Check sheet for the modelled part. Datum: model origin and axes. Units: mm. Coordinates: 2 decimals unless noted, no trailing zeros. Write each loop counter-clockwise with the first axis right and the second up, starting at its lowest first coordinate (ties: lowest second). Pieces come first, ordered by that corner, then holes. Notation, with made-up numbers: (-5, 71) - (9, 71) arc R25 cw to (9, 104) - close; hole circle Ø5 at (0, 67). An arc over 180 degrees is marked (long way). Use one line per item in the form item = value. Start each with the question number.
1. Cross-section at A-A on y = 0.25. Record the boundary of the cut face in (x, z).
2. Cross-section at B-B on y = -5. Record the boundary of the cut face in (x, z).
3. Scan lines: line 1 along Y through (x, z) = (-2, -45); line 2 along X through (y, z) = (3.75, -23); line 3 along X through (y, z) = (3.75, -35). Record each from-to range of solid material in increasing order.
4. Cross-section at C-C on y = 5.5. Record the boundary of the cut face in (x, z).
5. Go/stop test with flat-tipped pins: pin 1 Ø10 at (x, z) = (-1.5, -23.5) entering from -Y; pin 2 Ø2 at (y, z) = (-4, -29.5) entering from +X; pin 3 Ø3 at (y, z) = (-2.5, -75.5) entering from -X. Record where each tip stops, or that it passes through.
```python
from build123d import *

# Parameters (mm, degrees)
F1_DEPTH    = 6.35
F2_DEPTH    = 6.35
F4_DEPTH    = 25.4
F5_T1_DEPTH = 66.3794734437
F5_T3_DEPTH = 66.4252991911
F5_T5_DEPTH = 63.2525240866
F5_T7_DEPTH = 63.2028524021


# Not quite as in the source:
# - a fillet or chamfer that OpenCascade refuses, or shapes differently, is made with other operations: its cross-section is extruded or revolved along the edge and cut away or added


with BuildPart() as f1:
    # F0 (on Front) → F1 (new body)
    with BuildSketch(Plane.XZ):
        Polygon((10.5009634349, -8.6313571018), (0, -8.4001217037), (-10.5245159939, -8.168367669), (-8.3013391122, -91.856867075), (8.6683045514, -91.856867075), align=None)
    extrude(amount=F1_DEPTH)

    # F2 (add): a face of the model
    f2_faces = [f1.faces().sort_by_distance(p)[0] for p in [
        (0.0745348421, 0, -48.6438367355),
    ]]
    extrude(f2_faces, amount=F2_DEPTH)

    # F3 (on face) → F4 (cut)
    with BuildSketch(Plane.XZ.offset(6.35)):
        Polygon((7.741477061, -8.5705921125), (0, -12.6956291497), (-8.4089043082, -8.2149542811), (-10.5245159939, -8.168367669), (-10.4707083295, -10.1938847244), (0, -15.2933746576), (10.4665109394, -10.1959289555), (10.5009634349, -8.6313571018), align=None)
        Polygon((-8.4089043082, -8.2149542811), (0, -12.6956291497), (7.741477061, -8.5705921125), align=None)
        Polygon((0, -15.2933746576), (-10.4707083295, -10.1938847244), (-10.1647846318, -21.7099702861), (-2.6734457948, -26.4930181658), (-2.660532576, -26.5012629595), (-2.6115273083, -26.532551698), align=None)
        Polygon((10.2136542458, -21.6787681594), (10.4665109394, -10.1959289555), (0, -15.2933746576), (2.660532576, -26.5012629595), align=None)
        Polygon((-2.6734457948, -26.4930181658), (-10.1647846318, -21.7099702861), (-10.0923027152, -24.4384544155), (-3.4606218927, -28.9392464633), (-3.2699760565, -29.068634063), (-3.2102312503, -29.1091816943), (-2.6115273083, -26.532551698), (-2.660532576, -26.5012629595), align=None)
        Polygon((10.15380398, -24.3967147102), (10.2136542458, -21.6787681594), (2.660532576, -26.5012629595), (3.2699760565, -29.068634063), align=None)
        Polygon((-3.4606218927, -28.9392464633), (-10.0923027152, -24.4384544155), (-9.2748739024, -55.2094611118), (-3.2102312503, -29.1091816943), (-3.2699760565, -29.068634063), align=None)
        Polygon((9.4752950296, -55.2094611118), (10.15380398, -24.3967147102), (3.2699760565, -29.068634063), align=None)
        Polygon((-4.0967862529, -75.6694136894), (-9.2748739024, -55.2094611118), (-8.7972565245, -73.1887240187), (-4.2695118804, -75.5782571337), (-4.199302435, -75.6153104147), align=None)
        Polygon((9.0827017549, -73.0380792973), (9.4752950296, -55.2094611118), (4.199302435, -75.6153104147), align=None)
        Polygon((-3.1505538377, -79.4082206875), (-4.0967862529, -75.6694136894), (-4.199302435, -75.6153104147), (-4.2695118804, -75.5782571337), (-8.7972565245, -73.1887240187), (-8.7198462703, -76.1027287805), (-3.3105833326, -79.3132398248), (-3.2309755221, -79.3604887305), align=None)
        Polygon((9.0827017549, -73.0380792973), (4.199302435, -75.6153104147), (3.2309755221, -79.3604887305), (9.0191284413, -75.9250985328), align=None)
        Polygon((-0.965611629, -88.0414878319), (-3.1505538377, -79.4082206875), (-3.2309755221, -79.3604887305), (-3.3105833326, -79.3132398248), (-8.7198462703, -76.1027287805), (-8.5424459568, -82.7807246478), (-1.0061214638, -88.0133609601), (-0.9910429813, -88.023830283), align=None)
        Polygon((9.0191284413, -75.9250985328), (3.2309755221, -79.3604887305), (0.9910429813, -88.023830283), (8.8732221424, -82.5510594467), align=None)
        Polygon((0, -91.856867075), (-0.965611629, -88.0414878319), (-0.9910429813, -88.023830283), (-1.0061214638, -88.0133609601), (-8.5424459568, -82.7807246478), (-8.434321605, -86.8509202434), align=None)
        Polygon((8.8732221424, -82.5510594467), (0.9910429813, -88.023830283), (0, -91.856867075), (8.7830958233, -86.6439154273), align=None)
        Polygon((-8.3013391122, -91.856867075), (0, -91.856867075), (-8.434321605, -86.8509202434), align=None)
        Polygon((8.7830958233, -86.6439154273), (0, -91.856867075), (8.6683045514, -91.856867075), align=None)
    extrude(amount=-F4_DEPTH, mode=Mode.SUBTRACT)

    # F5: fillet of radius 5.08 on 8 edges, made by hand

    # F5_s2 → F5_t1 (cut)
    with BuildSketch(Plane(origin=(-15.5207879816, 0, -66.796500031), x_dir=(0, 1, 0), z_dir=(0.2263297481, 0, 0.9740507405))):
        with BuildLine():
            ThreePointArc((-6.35, -8.5413456341), (-4.8621024484, -4.9492431857), (-1.27, -3.4613456341))
            Line((-1.27, -3.4613456341), (-6.35, -3.4613456341))
            Line((-6.35, -3.4613456341), (-6.35, -8.5413456341))
        make_face()
        with BuildLine():
            ThreePointArc((6.35, -8.5413456341), (4.8621024484, -4.9492431857), (1.27, -3.4613456341))
            Line((1.27, -3.4613456341), (6.35, -3.4613456341))
            Line((6.35, -3.4613456341), (6.35, -8.5413456341))
        make_face()
    extrude(amount=F5_T1_DEPTH, mode=Mode.SUBTRACT)

    # F5_s4 → F5_t3 (cut)
    with BuildSketch(Plane(origin=(0.5034707355, 0, -2.1209451889), x_dir=(0, 1, 0), z_dir=(0.2309622408, 0, -0.9729627143))):
        with BuildLine():
            ThreePointArc((-1.27, -3.5321920799), (-4.8621024484, -5.0200896315), (-6.35, -8.6121920799))
            Line((-6.35, -8.6121920799), (-6.35, -3.5321920799))
            Line((-6.35, -3.5321920799), (-1.27, -3.5321920799))
        make_face()
        with BuildLine():
            ThreePointArc((1.27, -3.5321920799), (4.8621024484, -5.0200896315), (6.35, -8.6121920799))
            Line((6.35, -8.6121920799), (6.35, -3.5321920799))
            Line((6.35, -3.5321920799), (1.27, -3.5321920799))
        make_face()
    extrude(amount=F5_T3_DEPTH, mode=Mode.SUBTRACT)

    # F5_s6 → F5_t5 (cut)
    with BuildSketch(Plane(origin=(-9.6073030151, 0, -37.1579705651), x_dir=(0, 1, 0), z_dir=(-0.2503213526, 0, -0.9681628068))):
        with BuildLine():
            ThreePointArc((-6.35, 17.9137352141), (-4.8621024484, 21.5058376626), (-1.27, 22.9937352141))
            Line((-1.27, 22.9937352141), (-6.35, 22.9937352141))
            Line((-6.35, 22.9937352141), (-6.35, 17.9137352141))
        make_face()
        with BuildLine():
            ThreePointArc((1.27, 22.9937352141), (4.8621024484, 21.5058376626), (6.35, 17.9137352141))
            Line((6.35, 17.9137352141), (6.35, 22.9937352141))
            Line((6.35, 22.9937352141), (1.27, 22.9937352141))
        make_face()
    extrude(amount=F5_T5_DEPTH, mode=Mode.SUBTRACT)

    # F5_s8 → F5_t7 (cut)
    with BuildSketch(Plane(origin=(24.9640295189, 0, -98.6392843591), x_dir=(0, 1, 0), z_dir=(-0.2453485204, 0, 0.9694349403))):
        with BuildLine():
            ThreePointArc((-6.35, 17.4569464222), (-4.8621024484, 21.0490488706), (-1.27, 22.5369464222))
            Line((-1.27, 22.5369464222), (-6.35, 22.5369464222))
            Line((-6.35, 22.5369464222), (-6.35, 17.4569464222))
        make_face()
        with BuildLine():
            ThreePointArc((6.35, 17.4569464222), (4.8621024484, 21.0490488706), (1.27, 22.5369464222))
            Line((1.27, 22.5369464222), (6.35, 22.5369464222))
            Line((6.35, 22.5369464222), (6.35, 17.4569464222))
        make_face()
    extrude(amount=F5_T7_DEPTH, mode=Mode.SUBTRACT)


solid = f1.part
```
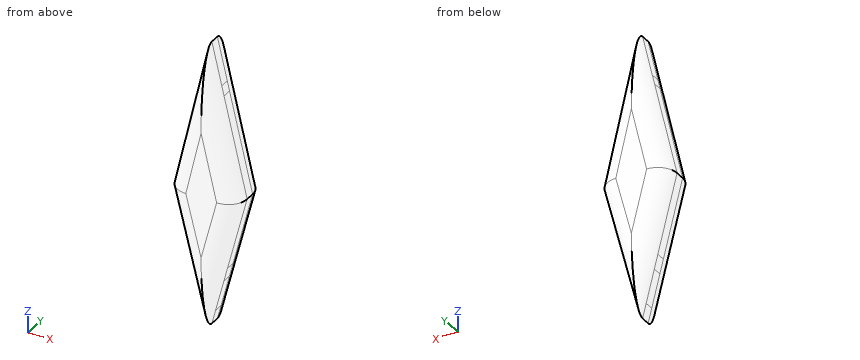
Final values:
q1.outline = (-9.27, -55.21) - (0, -91.86) - (9.48, -55.21) - (0, -15.29) - close
q2.outline = (-7.6, -55.19) - (0.02, -85.27) - (7.79, -55.19) - (0.02, -22.43) - close
q3.line_1 = -6.34 to 6.34
q3.line_2 = -1.13 to 1.16
q3.line_3 = -3.92 to 4.01
q4.outline = (-6.94, -55.19) - (0.02, -82.71) - (7.14, -55.19) - (0.02, -25.21) - close
q5.pin_1 = -5.89
q5.pin_2 = 3.13
q5.pin_3 = -4.45
